```python
from build123d import *

# Parameters (mm, degrees)
SKETCH_1_R          = 17.5
EXTRUDE_1_DEPTH     = 8
SKETCH_2_R          = 7
EXTRUDE_2_DEPTH     = 2.5
SKETCH_3_R          = 5
EXTRUDE_3_DEPTH     = 9.5
SKETCH_4_R          = 1.6
CUT_EXTRUDE_1_DEPTH = 28.504545079
SKETCH_5_R          = 3.5
SKETCH_5_R_2        = 1.6
CUT_EXTRUDE_2_DEPTH = 4


with BuildPart() as part:
    # ｽｹｯﾁ1 → ﾎﾞｽ - 押し出し1 (new body)
    with BuildSketch(Plane.XY):
        Circle(SKETCH_1_R)
    extrude(amount=EXTRUDE_1_DEPTH)

    # ｽｹｯﾁ2 → ﾎﾞｽ - 押し出し2 (add)
    with BuildSketch(Plane.XY.offset(8)):
        Circle(SKETCH_2_R)
    extrude(amount=EXTRUDE_2_DEPTH)

    # ｽｹｯﾁ3 → ﾎﾞｽ - 押し出し3 (add)
    with BuildSketch(Plane.XY.offset(10.5)):
        Circle(SKETCH_3_R)
    extrude(amount=EXTRUDE_3_DEPTH)

    # ｽｹｯﾁ4 → ｶｯﾄ - 押し出し1 (cut, through all)
    with BuildSketch(Plane.XY.offset(8)):
        with Locations((8.838834765, 8.838834765)):
            Circle(SKETCH_4_R)
        with Locations((8.838834765, -8.838834765)):
            Circle(SKETCH_4_R)
        with Locations((-8.838834765, -8.838834765)):
            Circle(SKETCH_4_R)
        with Locations((-8.838834765, 8.838834765)):
            Circle(SKETCH_4_R)
    extrude(amount=-CUT_EXTRUDE_1_DEPTH, mode=Mode.SUBTRACT)

    # ｽｹｯﾁ5 → ｶｯﾄ - 押し出し2 (cut)
    # profile 1 of 4: a face of its own
    with BuildSketch(Plane.XY.offset(8)):
        with Locations((8.838834765, 8.838834765)):
            Circle(SKETCH_5_R)
        with Locations((8.838834765, 8.838834765)):
            Circle(SKETCH_5_R_2, mode=Mode.SUBTRACT)
    # profile 2 of 4: a face of its own
    with BuildSketch(Plane.XY.offset(8)):
        with Locations((8.838834765, -8.838834765)):
            Circle(SKETCH_5_R)
        with Locations((8.838834765, -8.838834765)):
            Circle(SKETCH_5_R_2, mode=Mode.SUBTRACT)
    # profile 3 of 4: a face of its own
    with BuildSketch(Plane.XY.offset(8)):
        with Locations((-8.838834765, -8.838834765)):
            Circle(SKETCH_5_R)
        with Locations((-8.838834765, -8.838834765)):
            Circle(SKETCH_5_R_2, mode=Mode.SUBTRACT)
    # profile 4 of 4: a face of its own
    with BuildSketch(Plane.XY.offset(8)):
        with Locations((-8.838834765, 8.838834765)):
            Circle(SKETCH_5_R)
        with Locations((-8.838834765, 8.838834765)):
            Circle(SKETCH_5_R_2, mode=Mode.SUBTRACT)
    extrude(amount=-CUT_EXTRUDE_2_DEPTH, mode=Mode.SUBTRACT)


solid = part.part
```
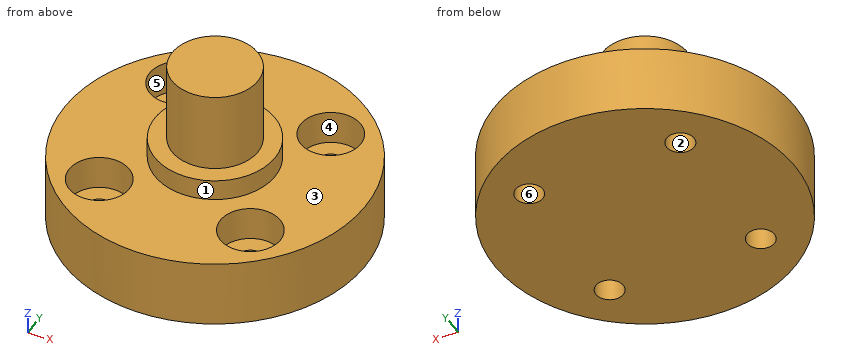
The listing builds one solid part. Answer for the finished solid, in the listing's coordinates (mm). Face numbers are marked on the shaded views. A direction names the side the tool comes from. Give positions to 0.01 mm unless a question says otherwise; leave off trailing zeros. Order: outer loops, then holes, each group sorted by start corner. A loop starts at its lowest first (then second) coordinate and runs counter-clockwise, first axis right, second up. Notation, with made-up numbers: (83.5, -15.5) - (120.5, -15.5) arc R27 ccw to (120.5, 4.5) - close; hole circle Ø7 at (-21, 5). An arc over 180 degrees is marked (long way). Use one line per item in the form item = value. Start each with the question number.
(1) A cutting plane is placed at B-B, the plane x = 8. Write down the section's boundary in (y, z).
(2) Flat-ended cylindrical pins translate along their axes: pin 1 Ø1.5 at (x, y) = (-9.5, -2.5) entering from -Z; pin 2 Ø8 at (x, y) = (-8.84, -8.84) entering from +Z; pin 3 Ø1 at (x, y) = (-6.5, 8.5) entering from +Z; pin 4 Ø12 at (x, z) = (8.5, 2.5) entering from +Y. Find the tip coordinate at first contact, or state that the pin passes through.
(3) A cutting plane is placed at A-A, the plane x = 0. Write down the section's boundary in (y, z).
(4) The mould has two halves that part along Y. Classify the marked faces 1, 2, 3 and 4: released by +Y, released by -Y, zero draft, split by the parting line, or undercut.
(5) For the marked faces 5 and 6, determine the directions among +Z, -Z, +X, -X, +Y, -Y from which every point of the face is accessible in a straight line to the end or side of a thin tool.
(6) Consider line 1 (Y direction, x = 9.5, z = 3); line 2 (X direction, y = 8, z = 6.5); line 3 (Z direction, x = -2, y = -7). Determine where each line is inside the solid, lowest interval first. Write a range as from..to.
(7) A cutting plane is placed at D-D, the plane z = 13.25. Write down the section's boundary in (x, y), then the cut area to 3 significant figures.
Ans:
q1.outline = (-15.56, 0) - (-10.2, 0) - (-10.2, 4) - (-12.24, 4) - (-12.24, 8) - (-15.56, 8) - close; (-7.48, 0) - (7.48, 0) - (7.48, 4) - (5.44, 4) - (5.44, 8) - (-5.44, 8) - (-5.44, 4) - (-7.48, 4) - close; (10.2, 0) - (15.56, 0) - (15.56, 8) - (12.24, 8) - (12.24, 4) - (10.2, 4) - close
q2.pin_1 = 0
q2.pin_2 = 8
q2.pin_3 = 4
q2.pin_4 = 17.32
q3.outline = (-17.5, 0) - (17.5, 0) - (17.5, 8) - (7, 8) - (7, 10.5) - (5, 10.5) - (5, 20) - (-5, 20) - (-5, 10.5) - (-7, 10.5) - (-7, 8) - (-17.5, 8) - close
q4.face_1 = split by the parting line
q4.face_2 = undercut
q4.face_3 = zero draft
q4.face_4 = undercut
q5.face_5 = +Z
q5.face_6 = +Z, -Z
q6.line_1 = -14.7..-10.3, -7.38..7.38, 10.3..14.7
q6.line_2 = -15.56..-12.24, -5.44..5.44, 12.24..15.56
q6.line_3 = 0..8
q7.outline = circle Ø10 at (0, 0)
q7.area = 78.5 mm^2
